Can you work these out from the model? Positions are in its coordinate system, mm. A direction names the side the tool comes from. Round coordinates to 2 decimals unless told otherwise and drop trailing zeros. Write each loop counter-clockwise with the first axis right and the second up, starting at its lowest first coordinate (ties: lowest second). Pieces come first, ordered by that corner, then holes.
Q1. I'm going to push flat-ended pins straight in: pin 1 Ø1 at (x, z) = (37, -11.5) entering from +Y; pin 2 Ø0.5 at (x, z) = (70.5, -6.5) entering from -Y; pin 3 Ø1.5 at (y, z) = (0.5, -25.5) entering from -X; pin 4 Ø4 at (y, z) = (2, -21.5) entering from +X. Where does each tip first touch, or does it pass through?
Q2. Please list where these lines run through material, in increasing order: line 1 along Z through (x, y) = (61.75, 7.5); line 2 along X through (y, z) = (-3, -27); line 3 along X through (y, z) = (16, -22.5).
Q3. If we section it at D-D (x = 47.5): Please give me the cut outline in (y, z), plus the area to 3 significant figures.
Q4. If we section it at A-A (z = -15): Please give me the cut outline in (x, y).
Q5. We'd pull the mould along X, two halves only. Please class faces 1 (the flat face through (39, -0.5, -15)), 2 (the flat face through (63.662, -13.14, -0.507)), 3 (the flat face through (25, 1, -22)): +X half, -X half, draft (parallel to the pull), parting line (faces both ways), or undercut.
Q6. If we section it at C-C (x = 24): Please give me the cut outline in (y, z).
Q7. For faces 4 (the flat face through (34, 1, -22)), 5 (the flat face through (29.437, 2.594, -23.673)), 6 (the flat face through (30, 1.5, -22)), 7 (the flat face through (64, 17.5, -15)), 8 (the flat face through (58.51, 14.62, -2.81)), which set-ups out of +Z, -Z, +X, -X, +Y, -Y let a thin tool reach every point of the face, with its end or its side?
from build123d import *

# Parameters (mm, degrees)
SKETCH084_W               = 50
SKETCH084_H               = 30
PAD025_DEPTH              = 25
PAD026_DEPTH              = 12.5
SKETCH086_R               = 2
POCKET054_DEPTH           = 6
SKETCH087_W               = 38
SKETCH087_H               = 30
POCKET055_DEPTH           = 18
SKETCH088_R               = 2
POCKET056_DEPTH           = 25.001
POCKET057_DEPTH           = 30.001
SKETCH090_R               = 3.15
POCKET058_DEPTH           = 50.001
SKETCH091_W               = 10
SKETCH091_H               = 8
PAD027_DEPTH              = 1
CHAMFER020_SIZE           = 5
CHAMFER021_SIZE           = 1
POCKET059_DEPTH           = 0.15
CHAMFER022_SIZE           = 0.4
CHAMFER023_SIZE           = 0.99
SKETCH142_W               = 9
SKETCH142_H               = 9
PAD043_DEPTH              = 5
CHAMFER009002001021_SIZE2 = 7
CHAMFER009002001021_SIZE  = 4.99
SKETCH143_W               = 3
SKETCH143_H               = 2
POCKET093_DEPTH           = 11.001
CHAMFER009002001022_SIZE  = 1


with BuildPart() as part:
    # Sketch084 → Pad025 (new body)
    with BuildSketch(Plane.XZ):
        with Locations((25, 15)):
            Rectangle(SKETCH084_W, SKETCH084_H)
    extrude(amount=PAD025_DEPTH)

    # Sketch085 (on Face6 of Pad025) → Pad026 (join)
    with BuildSketch(Plane.XZ.offset(25)):
        Polygon((0.180278, 30), (8.15, 18.045416), (8.15, 11.954584), (0.180278, 0), (50, 0), (50, 30), align=None)
    extrude(amount=PAD026_DEPTH)

    # Sketch086 (on Face4 of Pad026) → Pocket054 (cut)
    with BuildSketch(Plane(origin=(0, 0, 0), x_dir=(1, 0, 0), z_dir=(0, 1, 0))):
        with Locations((4, -15)):
            Circle(SKETCH086_R)
    extrude(amount=-POCKET054_DEPTH, mode=Mode.SUBTRACT)

    # Sketch087 (on Face4 of Pocket054) → Pocket055 (cut)
    with BuildSketch(Plane(origin=(0, 0, 0), x_dir=(1, 0, 0), z_dir=(0, 1, 0))):
        with Locations((19, -15)):
            Rectangle(SKETCH087_W, SKETCH087_H)
    extrude(amount=-POCKET055_DEPTH, mode=Mode.SUBTRACT)

    # Sketch088 (on Face7 of Pocket055) → Pocket056 (cut, through all)
    with BuildSketch(Plane.XZ.offset(25)):
        with Locations((4, 15)):
            Circle(SKETCH088_R)
    extrude(amount=-POCKET056_DEPTH, mode=Mode.SUBTRACT)

    # Sketch089 (on Face13 of Pocket056) → Pocket057 (cut, through all)
    with BuildSketch(Plane(origin=(0, 0, 30), x_dir=(-1, 0, 0), z_dir=(0, 0, 1))):
        Polygon((-50, 37.5), (-37.5, 37.5), (-50, 25), align=None)
    extrude(amount=-POCKET057_DEPTH, mode=Mode.SUBTRACT)

    # Sketch090 (on Face11 of Pocket057) → Pocket058 (cut, through all)
    with BuildSketch(Plane(origin=(50, 0, 0), x_dir=(0, 0, 1), z_dir=(1, 0, 0))):
        with Locations((15, 10)):
            Circle(SKETCH090_R)
    extrude(amount=-POCKET058_DEPTH, mode=Mode.SUBTRACT)

    # Sketch091 (on Face11 of Pocket058) → Pad027 (join)
    with BuildSketch(Plane(origin=(50, 0, 0), x_dir=(0, 0, 1), z_dir=(1, 0, 0))):
        with Locations((5, 10)):
            Rectangle(SKETCH091_W, SKETCH091_H)
        with Locations((25, 10)):
            Rectangle(SKETCH091_W, SKETCH091_H)
    extrude(amount=PAD027_DEPTH)

    # Chamfer020
    chamfer020_edges = [part.edges().sort_by_distance(p)[0] for p in [
        (44, 0, 30),
        (44, 0, 0),
    ]]
    chamfer(chamfer020_edges, length=CHAMFER020_SIZE)

    # Chamfer021
    chamfer021_edges = [part.edges().sort_by_distance(p)[0] for p in [
        (18.840139, -37.5, 30),
        (4.165139, -37.5, 24.022708),
        (8.15, -37.5, 15),
        (18.840139, -37.5, 0),
        (43.75, -31.25, 30),
        (43.75, -31.25, 0),
        (0.180278, -31.25, 0),
        (0.180278, -31.25, 30),
        (19, -18, 30),
        (38, -11.5, 30),
        (38, -2.5, 27.5),
        (38, 0, 15),
        (38, -2.5, 2.5),
        (38, -11.5, 0),
        (19, -18, 0),
        (4.165139, -37.5, 5.977292),
    ]]
    chamfer(chamfer021_edges, length=CHAMFER021_SIZE)

    # Chamfer021 Face21 → Pocket059 (cut)
    with BuildSketch(Plane(origin=(0, -21.515152, 15), x_dir=(0, 1, 0), z_dir=(-1, 0, 0))):
        Polygon((3.515152, -14), (3.515152, 14), (2.515152, 15), (-3.484848, 15), (-3.484848, -15), (2.515152, -15), align=None)
    extrude(amount=-POCKET059_DEPTH, mode=Mode.SUBTRACT)

    # Chamfer022
    chamfer022_edges = [part.edges().sort_by_distance(p)[0] for p in [
        (38, -10, 11.85),
        (2, -18, 15),
    ]]
    chamfer(chamfer022_edges, length=CHAMFER022_SIZE)

    # Chamfer023
    chamfer023_edges = [part.edges().sort_by_distance(p)[0] for p in [
        (51, -10, 0),
        (51, -10, 20),
    ]]
    chamfer(chamfer023_edges, length=CHAMFER023_SIZE)

    # Sketch142 (on Face34 of Chamfer023) → Pad043 (join)
    with BuildSketch(Plane(origin=(0, -18, 0), x_dir=(1, 0, 0), z_dir=(0, 1, 0))):
        with Locations((9.5, -6.5)):
            Rectangle(SKETCH142_W, SKETCH142_H)
    extrude(amount=PAD043_DEPTH)

    # Chamfer009002001021
    chamfer009002001021_edges = [part.edges().sort_by_distance(p)[0] for p in [
        (9.5, -13, 2),
    ]]
    chamfer009002001021_side = part.faces().sort_by_distance((9.5, -15.5, 2))[0]
    chamfer(chamfer009002001021_edges, length=CHAMFER009002001021_SIZE, length2=CHAMFER009002001021_SIZE2, reference=chamfer009002001021_side)

    # Sketch143 (on Face7 of Chamfer009002001021) → Pocket093 (cut, through all)
    with BuildSketch(Plane(origin=(0, 0, 11), x_dir=(-1, 0, 0), z_dir=(0, 0, 1))):
        with Locations((-9.5, 17)):
            Rectangle(SKETCH143_W, SKETCH143_H)
    extrude(amount=-POCKET093_DEPTH, mode=Mode.SUBTRACT)

    # Chamfer009002001022
    chamfer009002001022_edges = [part.edges().sort_by_distance(p)[0] for p in [
        (9.5, -16, 11),
        (9.5, -16, 4.791583),
    ]]
    chamfer(chamfer009002001022_edges, length=CHAMFER009002001022_SIZE)


with BuildPart() as part_1:
    # Body009 placement: moved
    add(part.part.moved(Location((20, 17.5, -30))))


solid = part_1.part
A:
1. pin 1: stops at y = -0.5
1. pin 2: stops at y = 3.5
1. pin 3: stops at x = 25
1. pin 4: stops at x = 71
2. line 1: z = -30 to -18.15, -11.85 to 0
2. line 2: x = 20.15 to 70
2. line 3: x = 58 to 70
3. outline: (-20, -29) - (-19, -30) - (-1.5, -30) - (-0.5, -29) - (-0.5, -1) - (-1.5, 0) - (-19, 0) - (-20, -1) - close
3. area: 583 mm2
4. outline: (20.15, -7.5) - (22, -7.5) - (22, -0.9) - (21.6, -0.5) - (20.15, -0.5) - close; (26, -7.5) - (28.15, -7.5) - (28.15, -19) - (29.15, -20) - (57.5, -20) - (70, -7.5) - (70, 4.35) - (58.4, 4.35) - (58, 3.95) - (58, -0.5) - (26.4, -0.5) - (26, -0.9) - close; (58, 11.05) - (58.4, 10.65) - (70, 10.65) - (70, 17.5) - (59, 17.5) - (58, 16.5) - close
5. face 1: undercut
5. face 2: +X half
5. face 3: -X half
6. outline: (-20, -29) - (-19, -30) - (-1.5, -30) - (-0.5, -29) - (-0.5, -17.4) - (-0.9, -17) - (-7.5, -17) - (-7.5, -24.27) - (-19, -24.27) - (-20, -26.07) - close; (-20, -3.93) - (-19, -5.73) - (-7.5, -5.73) - (-7.5, -13) - (-0.9, -13) - (-0.5, -12.6) - (-0.5, -1) - (-1.5, 0) - (-19, 0) - (-20, -1) - close
7. face 4: +Z, -Z, +Y
7. face 5: -Z, -X, +Y
7. face 6: +Z, -Z
7. face 7: +Z, -Z, +X, -X, +Y
7. face 8: +Z, -X, +Y
